Can you work these out from the model? Positions are in its coordinate system, mm. A direction names the side the tool comes from. Give positions to 0.01 mm unless a question says otherwise; leave off trailing zeros. Write each loop counter-clockwise with the first axis right and the second up, starting at its lowest first coordinate (ties: lowest second). Pieces come first, ordered by that corner, then holes.
```python
from build123d import *

# Parameters (mm, degrees)
SKETCH_1_W      = 19
SKETCH_1_H      = 38
EXTRUDE_1_DEPTH = 3
EXTRUDE_2_DEPTH = 25
SKETCH_5_W      = 25
SKETCH_5_H      = 9.8
EXTRUDE_3_DEPTH = 2.5
CHAMFER_1_SIZE  = 2
FILLET_2_R      = 5
FILLET_3_R      = 1
FILLET_4_R      = 1


# Some blends are built 0.0001 mm under size
with BuildPart() as part:
    # 草图1 → 凸台-拉伸1 (new body)
    with BuildSketch(Plane.XY):
        Rectangle(SKETCH_1_W, SKETCH_1_H)
    extrude(amount=EXTRUDE_1_DEPTH)

    # 草图2 → 凸台-拉伸2 (add)
    with BuildSketch(Plane(origin=(0, 0, 0), x_dir=(-1, 0, 0), z_dir=(0, 0, -1))):
        Polygon((-9.5, 19), (9.5, 19), (9.5, -19), (-9.5, -19), (-9.5, -15), (5.5, -15), (5.5, 15), (-9.5, 15), align=None)
    extrude(amount=EXTRUDE_2_DEPTH)

    # 草图5 → 凸台-拉伸3 (add)
    with BuildSketch(Plane(origin=(9.5, 0, 0), x_dir=(0, 0, -1), z_dir=(1, 0, 0))):
        with Locations((12.5, 10.1)):
            Rectangle(SKETCH_5_W, SKETCH_5_H)
        with Locations((12.5, -10.1)):
            Rectangle(SKETCH_5_W, SKETCH_5_H)
    extrude(amount=-EXTRUDE_3_DEPTH)

    # 倒角1
    chamfer_1_edges = [part.edges().sort_by_distance(p)[0] for p in [
        (8.25, 5.2, -25),
        (8.25, -5.2, -25),
    ]]
    chamfer(chamfer_1_edges, length=CHAMFER_1_SIZE)

    # 圆角2
    # the kernel refuses this fillet: 5 mm, written as the material it takes off along each edge
    with BuildSketch(Plane(origin=(4.5, -14, -2), x_dir=(0, -1, 0), z_dir=(1, 0, 0))) as fillet_2_piece_1_section:
        Polygon((0, 0), (FILLET_2_R, 0), (FILLET_2_R, -FILLET_2_R), (0, -FILLET_2_R), align=None)
    fillet_2_piece_1 = extrude(amount=FILLET_2_R, mode=Mode.PRIVATE)
    fillet_2_piece_1 = fillet_2_piece_1 - Plane(origin=(4.5, -14, -2), x_dir=(0, 0.7071067811865475, -0.7071067811865475), z_dir=(1, 0, 0)) * Sphere(FILLET_2_R, mode=Mode.PRIVATE)
    add(fillet_2_piece_1, mode=Mode.SUBTRACT)
    with BuildSketch(Plane(origin=(-4.5, -14, -2), x_dir=(0, -1, 0), z_dir=(-1, 0, 0))) as fillet_2_piece_2_section:
        Polygon((0, 0), (FILLET_2_R, 0), (FILLET_2_R, FILLET_2_R), (0, FILLET_2_R), align=None)
    fillet_2_piece_2 = extrude(amount=FILLET_2_R, mode=Mode.PRIVATE)
    fillet_2_piece_2 = fillet_2_piece_2 - Plane(origin=(-4.5, -14, -2), x_dir=(0, 0.7071067811865475, -0.7071067811865475), z_dir=(-1, 0, 0)) * Sphere(FILLET_2_R, mode=Mode.PRIVATE)
    add(fillet_2_piece_2, mode=Mode.SUBTRACT)
    with BuildSketch(Plane(origin=(-4.5, 14, -2), x_dir=(-1, 0, 0), z_dir=(0, 0, 1))) as fillet_2_piece_3_section:
        Polygon((0, 0), (FILLET_2_R, 0), (FILLET_2_R, -FILLET_2_R), (0, -FILLET_2_R), align=None)
    fillet_2_piece_3 = extrude(amount=FILLET_2_R, mode=Mode.PRIVATE)
    fillet_2_piece_3 = fillet_2_piece_3 - Plane(origin=(-4.5, 14, -2), x_dir=(0.7071067811865476, -0.7071067811865475, 0), z_dir=(0, 0, 1)) * Sphere(FILLET_2_R, mode=Mode.PRIVATE)
    add(fillet_2_piece_3, mode=Mode.SUBTRACT)
    with BuildSketch(Plane(origin=(4.5, 14, -2), x_dir=(0, 0, 1), z_dir=(1, 0, 0))) as fillet_2_piece_4_section:
        Polygon((0, 0), (FILLET_2_R, 0), (FILLET_2_R, -FILLET_2_R), (0, -FILLET_2_R), align=None)
    fillet_2_piece_4 = extrude(amount=FILLET_2_R, mode=Mode.PRIVATE)
    fillet_2_piece_4 = fillet_2_piece_4 - Plane(origin=(4.5, 14, -2), x_dir=(0, -0.7071067811865475, -0.7071067811865475), z_dir=(1, 0, 0)) * Sphere(FILLET_2_R, mode=Mode.PRIVATE)
    add(fillet_2_piece_4, mode=Mode.SUBTRACT)
    with BuildSketch(Plane(origin=(9.5, -19, -2), x_dir=(0, 1, 0), z_dir=(0, 0, -1))) as fillet_2_piece_5:
        with BuildLine():
            CenterArc((FILLET_2_R, -FILLET_2_R), FILLET_2_R, 90, 90)
            Line((0, -FILLET_2_R), (0, 0))
            Line((0, 0), (FILLET_2_R, 0))
        make_face()
    extrude(amount=35.5, mode=Mode.SUBTRACT)
    with BuildSketch(Plane(origin=(-22, -19, -25), x_dir=(0, 1, 0), z_dir=(1, 0, 0)), Plane(origin=(22, 19, -25), x_dir=(0, -1, 0), z_dir=(-1, 0, 0))) as fillet_2_piece_6:
        with BuildLine():
            CenterArc((FILLET_2_R, FILLET_2_R), FILLET_2_R, 180, 90)
            Line((0, FILLET_2_R), (0, 0))
            Line((0, 0), (FILLET_2_R, 0))
        make_face()
    extrude(amount=44, mode=Mode.SUBTRACT)
    with BuildSketch(Plane(origin=(4.5, -19, 3), x_dir=(0, 0, -1), z_dir=(-1, 0, 0)), Plane(origin=(-4.5, 19, 3), x_dir=(0, 0, -1), z_dir=(1, 0, 0))) as fillet_2_piece_7:
        with BuildLine():
            CenterArc((FILLET_2_R, -FILLET_2_R), FILLET_2_R, 90, 90)
            Line((0, -FILLET_2_R), (0, 0))
            Line((0, 0), (FILLET_2_R, 0))
        make_face()
    extrude(amount=9, mode=Mode.SUBTRACT)
    with BuildSketch(Plane(origin=(-9.5, -19, -37.5), x_dir=(1, 0, 0), z_dir=(0, 0, 1)), Plane(origin=(-9.5, 19, -37.5), x_dir=(0, -1, 0), z_dir=(0, 0, 1)), Plane(origin=(9.5, 19, -2), x_dir=(0, -1, 0), z_dir=(0, 0, -1))) as fillet_2_piece_8:
        with BuildLine():
            CenterArc((FILLET_2_R, FILLET_2_R), FILLET_2_R, 180, 90)
            Line((0, FILLET_2_R), (0, 0))
            Line((0, 0), (FILLET_2_R, 0))
        make_face()
    extrude(amount=35.5, mode=Mode.SUBTRACT)
    with BuildSketch(Plane(origin=(-9.5, -14, 3), x_dir=(0, 0, -1), z_dir=(0, 1, 0)), Plane(origin=(9.5, 14, 3), x_dir=(0, 0, -1), z_dir=(0, -1, 0))) as fillet_2_piece_9:
        with BuildLine():
            CenterArc((FILLET_2_R, -FILLET_2_R), FILLET_2_R, 90, 90)
            Line((0, -FILLET_2_R), (0, 0))
            Line((0, 0), (FILLET_2_R, 0))
        make_face()
    extrude(amount=28, mode=Mode.SUBTRACT)

    # 圆角3
    fillet_3_edges = [part.edges().sort_by_distance(p)[0] for p in [
        (-7.730244537, 17.816480084, -23.230244537),
        (-7.730244537, -17.816480084, -23.230244537),
        (-9.5, 0, -25),
    ]]
    fillet(fillet_3_edges, radius=FILLET_3_R)

    # 圆角4
    fillet_4_edges = [part.edges().sort_by_distance(p)[0] for p in [
        (9.394531565, 5.2, -0.978451782),
        (9.394531565, -5.2, -0.978451782),
        (8.035533906, 17.535533906, -23.535533906),
        (8.035533906, -17.535533906, -23.535533906),
        (9.5, -10.6, -25),
        (9.5, -5.2, -12.5),
        (9.5, 5.2, -12.5),
        (9.5, 10.6, -25),
    ]]
    fillet(fillet_4_edges, radius=FILLET_4_R - 0.0001)  # a hair under: the kernel refuses the full size


solid = part.part
```
1) Please list where these lines run through material, in increasing order: L1, parallel to Y at x = -0.5, z = -6.5; L2, parallel to X at y = 11, z = -17.75; L3, parallel to Z at x = -1.75, y = -8.
Values follow:
L1: y = -19 to -15, 15 to 19
L2: x = -9.5 to -5.5, 7 to 9.5
L3: z = 0 to 3
2) For faces 1 (the face through (-8, 17.57, -13.15)), 2 (the face through (8.3, -6.2, -24)), 3 (the face through (7, -10, -12)), which set-ups out of +Z, -Z, +X, -X, +Y, -Y let a thin tool reach every point of the face, with its end or its side?
Values follow:
face 1: +Z, -Z, -X, +Y
face 2: -Z, +X
face 3: -Z
3) For pin 1 Ø0.5 at (x, z) = (8, -6) entering from +Y; pin 2 Ø10 at (x, z) = (6, -5.5) entering from +Y; pin 3 Ø0.8 at (x, z) = (8, -9) entering from -Y; pin 4 Ø3 at (x, y) = (-3.5, 9) entering from -Z, each with a flat end and sliding along its axis, tell me the tip position at first contact or that it passes through.
Values follow:
pin 1: stops at y = 17.8
pin 2: stops at y = 19
pin 3: stops at y = -17.92
pin 4: stops at z = 0
4) Suppose I cut it at D-D on y = -9. Write out the boundary of the cut face in (x, z).
Values follow:
outline: (-9.5, -24) arc R1 ccw to (-8.5, -25) - (-5.5, -25) - (-5.5, 0) - (7, 0) - (7, -25) - (8.5, -25) arc R1 ccw to (9.5, -24) - (9.5, -2) arc R5 ccw to (4.5, 3) - (-4.5, 3) arc R5 ccw to (-9.5, -2) - close
5) Suppose I cut it at B-B on x = 0. Write out the boundary of the cut face in (y, z).
Values follow:
outline: (-19, -20) arc R5 ccw to (-15, -24.9) - (-15, 0) - (15, 0) - (15, -24.9) arc R5 ccw to (19, -20) - (19, -2) arc R5 ccw to (14, 3) - (-14, 3) arc R5 ccw to (-19, -2) - close
6) Suppose I cut it at A-A on y = -2.5. Write out the boundary of the cut face in (x, z).
Values follow:
outline: (-9.5, -24) arc R1 ccw to (-8.5, -25) - (-5.5, -25) - (-5.5, 0) - (9.08, 0) arc R5 ccw to (4.5, 3) - (-4.5, 3) arc R5 ccw to (-9.5, -2) - close
7) If we mould it in two halves opening along Y, with no side actions, what happens to faces 4 (the face through (8, 5.2, -11)), 5 (the face through (-9.199, 0.196, -24.715)), 6 (the face through (-5.5, 0, -12)), 7 (the face through (8, 17.57, -12.85))? For each: +Y half, -Y half, draft (parallel to the pull), parting line (faces both ways), or undercut.
Values follow:
face 4: undercut
face 5: draft
face 6: undercut
face 7: +Y half
8) Suppose I cut it at C-C on z = -13.5. Write out the boundary of the cut face in (x, y), plus the area to 3 significant figures.
Values follow:
outline: (-9.5, -14) arc R5 ccw to (-4.5, -19) - (4.5, -19) arc R5 ccw to (9.5, -14) - (9.5, -6.2) arc R1 ccw to (8.5, -5.2) - (7, -5.2) - (7, -15) - (-5.5, -15) - (-5.5, 15) - (7, 15) - (7, 5.2) - (8.5, 5.2) arc R1 ccw to (9.5, 6.2) - (9.5, 14) arc R5 ccw to (4.5, 19) - (-4.5, 19) arc R5 ccw to (-9.5, 14) - close
area: 299 mm2
